For this review, use the dimensioned drawing (mm, ordinates from the lowest corner) and the shaded views. A direction names the side the tool comes from. Round coordinates to 2 decimals unless told otherwise and drop trailing zeros. Write each loop counter-clockwise with the first axis right and the second up, starting at its lowest first coordinate (ties: lowest second). Pieces come first, ordered by that corner, then holes. Notation, with made-up numbers: M -19.5,-2 L 34.5,-2 A29 cw 34.5,27 Z; hole C 5.25,-6.75 d6. An arc over 180 degrees is marked long. Use one line per item in the form item = value. Start each with the question number.
Item 1: For the marked faces 1, 2 and 3, list the 3-axis set-ups (+Z, -Z, +X, -X, +Y, -Y) from which the entire face can be reached by the end or side of a thin tool; tool diameter is ignored.
Item 2: Add section B-B (x = 9.25). State the section outline as (y, z) points.
Item 3: Add section A-A (y = 46.5). State the section outline as (x, z) points.
Item 4: For P1, Ø3, axis at x = 9.5, y = 9, coming from the -Z side; P2, Ø4.5, axis at x = 9, z = 14.5, coming from the -Y side, all flat-tipped, find the tip position at first contact; note any pin that passes through.
Item 5: Draft analysis for pull direction X (two halves, no side actions). For the marked faces 4, 5 and 6, state which applies: released by +X, released by -X, zero draft, split by the parting line, or undercut.
Item 6: For line 1 (X direction, y = 27.5, z = 1.75); line 2 (Z direction, x = 9.75, y = 36); line 3 (Y direction, x = 9.75, z = 12), list the stretches that pass through material, from the lowest coordinate up. Write a range as [from, to].
Item 7: Add section C-C (z = 11). State the section outline as (x, y) points.
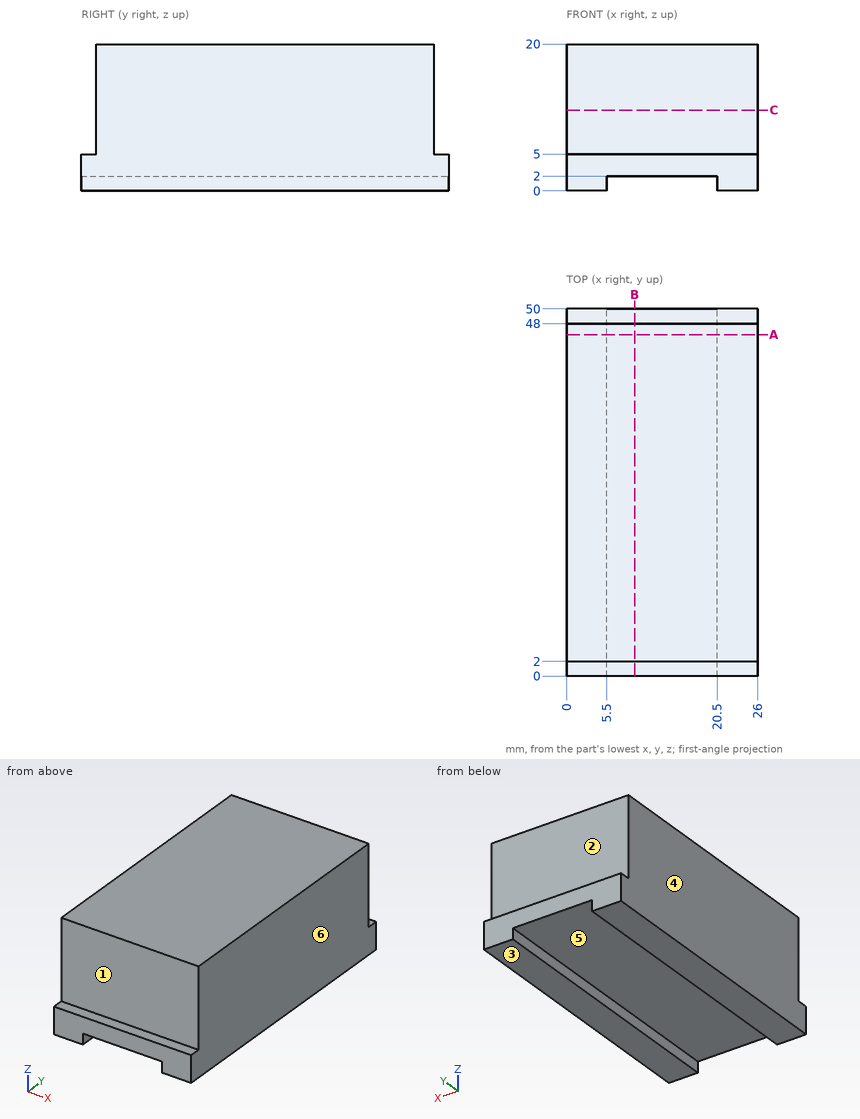
Calculated:
q1.face_1 = +Z, +X, -X, -Y
q1.face_2 = +Z, +X, -X, +Y
q1.face_3 = -Z, +X, -X, +Y, -Y
q2.outline = M 0,2 L 50,2 L 50,5 L 48,5 L 48,20 L 2,20 L 2,5 L 0,5 Z
q3.outline = M 0,0 L 5.5,0 L 5.5,2 L 20.5,2 L 20.5,0 L 26,0 L 26,20 L 0,20 Z
q4.P1 = 2
q4.P2 = 2
q5.face_4 = released by -X
q5.face_5 = undercut
q5.face_6 = released by +X
q6.line_1 = [0, 5.5], [20.5, 26]
q6.line_2 = [2, 20]
q6.line_3 = [2, 48]
q7.outline = M 0,2 L 26,2 L 26,48 L 0,48 Z
